Source: CAD feature listing. Evaluate the final solid. Frame: model axes, mm. Face numbers are marked on the shaded views. A direction names the side the tool comes from. Give positions to 0.01 mm unless a question says otherwise; leave off trailing zeros. Order: outer loops, then holes, each group sorted by start corner. A loop starts at its lowest first (then second) coordinate and runs counter-clockwise, first axis right, second up.
from build123d import *

# Parameters (mm, degrees)
F1_DEPTH  = 25.4
F2_R      = 6.9358016154
F2_R_2    = 6.6322643692
F3_DEPTH  = 13.2470994646
F5_DEPTH  = 44.5399002562
F6_R      = 5.3858777777
F7_DEPTH  = 44.5399002562
F9_DEPTH  = 13.2470994646
F11_DEPTH = 13.2470994646


with BuildPart() as f1:
    # F0 (on Front) → F1 (new body)
    with BuildSketch(Plane.XZ):
        Polygon((0, 13.2460994646), (0, 0), (76.1873051524, 0), (76.1873051524, 13.2460994646), (44.5389002562, 13.2460994646), (44.5389002562, 34.0486988425), (24.6252994984, 34.0486988425), (24.6252994984, 13.2460994646), align=None)
    extrude(amount=F1_DEPTH)

    # F2 (on face) → F3 (cut, through all)
    with BuildSketch(Plane.XY.offset(13.2460994646)):
        with Locations((12.0889488608, -12.7)):
            Circle(F2_R)
        with Locations((58.5328303277, -12.590335682)):
            Circle(F2_R_2)
    extrude(amount=-F3_DEPTH, mode=Mode.SUBTRACT)

    # F4 (on face) → F5 (cut, through all)
    with BuildSketch(Plane.YZ.offset(44.5389002562)):
        with BuildLine():
            ThreePointArc((-25.4, 23.6473991536), (-21.0511599992, 31.0022821178), (-13.0682997406, 34.0486988425))
            Line((-13.0682997406, 34.0486988425), (-25.4, 34.0486988425))
            Line((-25.4, 34.0486988425), (-25.4, 23.6473991536))
        make_face()
        with BuildLine():
            ThreePointArc((-12.3317002594, 34.0486988425), (-4.3488400008, 31.0022821178), (0, 23.6473991536))
            Line((0, 23.6473991536), (0, 34.0486988425))
            Line((0, 34.0486988425), (-12.3317002594, 34.0486988425))
        make_face()
    extrude(amount=-F5_DEPTH, mode=Mode.SUBTRACT)

    # F6 (on face) → F7 (cut, through all)
    with BuildSketch(Plane.YZ.offset(44.5389002562)):
        with Locations((-12.3317002594, 24.269701913)):
            Circle(F6_R)
    extrude(amount=-F7_DEPTH, mode=Mode.SUBTRACT)

    # F8 (on face) → F9 (cut, through all)
    with BuildSketch(Plane.XY.offset(13.2460994646)):
        with BuildLine():
            ThreePointArc((12.3126497492, -25.4), (0.2620769816, -12.7), (12.3126497492, 0))
            Line((12.3126497492, 0), (0, 0))
            Line((0, 0), (0, -25.4))
            Line((0, -25.4), (12.3126497492, -25.4))
        make_face()
    extrude(amount=-F9_DEPTH, mode=Mode.SUBTRACT)

    # F10 (on face) → F11 (cut, through all)
    with BuildSketch(Plane.XY.offset(13.2460994646)):
        with BuildLine():
            ThreePointArc((66.3337183287, 0), (72.8118717617, -3.7197458837), (76.1873051524, -10.383786007))
            Line((76.1873051524, -10.383786007), (76.1873051524, 0))
            Line((76.1873051524, 0), (66.3337183287, 0))
        make_face()
        with BuildLine():
            ThreePointArc((76.1873051524, -15.016213993), (72.8118717617, -21.6802541163), (66.3337183287, -25.4))
            Line((66.3337183287, -25.4), (76.1873051524, -25.4))
            Line((76.1873051524, -25.4), (76.1873051524, -15.016213993))
        make_face()
    extrude(amount=-F11_DEPTH, mode=Mode.SUBTRACT)


solid = f1.part
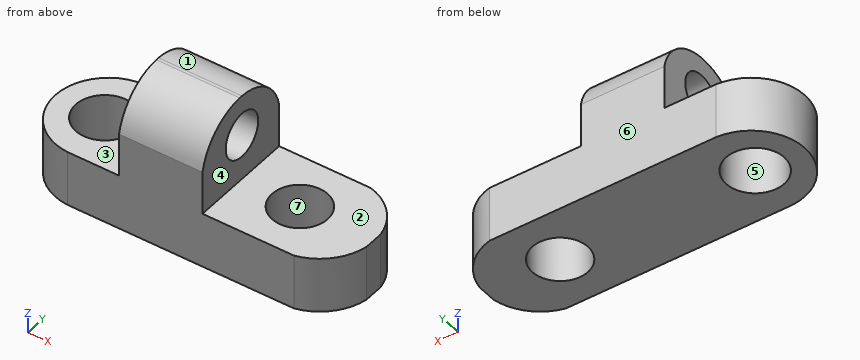
1) Pull-direction query (X, two-part tool) for the marked faces 4, 5, 6 and 7; classes: +X half, -X half, draft (parallel to the pull), parting line (faces both ways), or undercut.
Checks:
face 4: +X half
face 5: undercut
face 6: draft
face 7: undercut
2) Section query C-C on z = 5.5. Output: boundary loops of the cut face in (x, y) (1 decimal), and give its area (3 significant figures).
Checks:
outline: (12.3, -25.4) - (66.3, -25.4) arc R13 ccw to (76.2, -15) - (76.2, -10.4) arc R13 ccw to (66.3, 0) - (12.3, 0) arc R12.7 ccw to start; hole circle Ø13.9 at (12.1, -12.7); hole circle Ø13.3 at (58.5, -12.6)
area: 1,510 mm2
3) First-contact query: pin 1 Ø6 at (y, z) = (-3.5, 17) entering from -X; pin 2 Ø3 at (x, y) = (22, -13) entering from +Z; pin 3 Ø6 at (y, z) = (-7, 22) entering from +X; pin 4 Ø8.5 at (y, z) = (-12.33, 24.27) entering from -X. Flat tips, straight axial feed; report the tip coordinate or a pass-through.
Checks:
pin 1: stops at x = 24.63
pin 2: stops at z = 13.25
pin 3: stops at x = 44.54
pin 4: passes through
4) Section query B-B on z = 20.5. Output: boundary loops of the cut face in (x, y) (3 decimals), and give its area (3 significant figures).
Checks:
outline: (24.625, -25.4) - (44.539, -25.4) - (44.539, -16.178) - (24.625, -16.178) - close; (24.625, -8.485) - (44.539, -8.485) - (44.539, 0) - (24.625, 0) - close
area: 353 mm2
5) Ray query, L1, parallel to X at y = -7.25, z = 13; L2, parallel to X at y = -8, z = 12; L3, parallel to Z at x = 71.5, y = -22.25. Return the intervals inside material, ascending.
Checks:
L1: x = 1.49 to 7.8, 16.38 to 54.6, 62.47 to 75.2
L2: x = 1.16 to 6.99, 17.19 to 53.75, 63.32 to 75.52
L3: z = 0 to 13.25
6) Section query D-D on x = 37. Output: boundary loops of the cut face in (y, z), and give its area (3 significant figures).
Checks:
outline: (-25.4, 0) - (0, 0) - (0, 23.65) arc R12.95 ccw to (-12.33, 34.05) - (-13.07, 34.05) arc R12.95 ccw to (-25.4, 23.65) - close; hole circle Ø10.77 at (-12.33, 24.27)
area: 708 mm2
7) Section query A-A on x = 10.5. Output: boundary loops of the cut face in (y, z).
Checks:
outline: (-25.17, 0) - (-19.45, 0) - (-19.45, 13.25) - (-25.17, 13.25) - close; (-5.95, 0) - (-0.23, 0) - (-0.23, 13.25) - (-5.95, 13.25) - close
8) Reachability of the marked faces 1, 2 and 3 from +Z, -Z, +X, -X, +Y, -Y: full face, straight path, thin tool, end or side. Return the list, or none.
Checks:
face 1: +Z, +X, -X, +Y
face 2: +Z, +X, +Y, -Y
face 3: +Z, -X, +Y, -Y
